Source: three-view drawing plus pictorial views. Frame: mm from the lowest corner of the part. A direction names the side the tool comes from. Give positions to 0.01 mm unless a question says otherwise; leave off trailing zeros. Order: outer loops, then holes, each group sorted by start corner. A loop starts at its lowest first (then second) coordinate and runs counter-clockwise, first axis right, second up. Notation, with made-up numbers: (26, 89.5) -> (49, 89.5) arc R35 ccw to (49, 125.5) -> close; hole circle Ø5 at (-37, 43). An arc over 180 degrees is marked (long way). Answer in a Markdown table with one row per item.
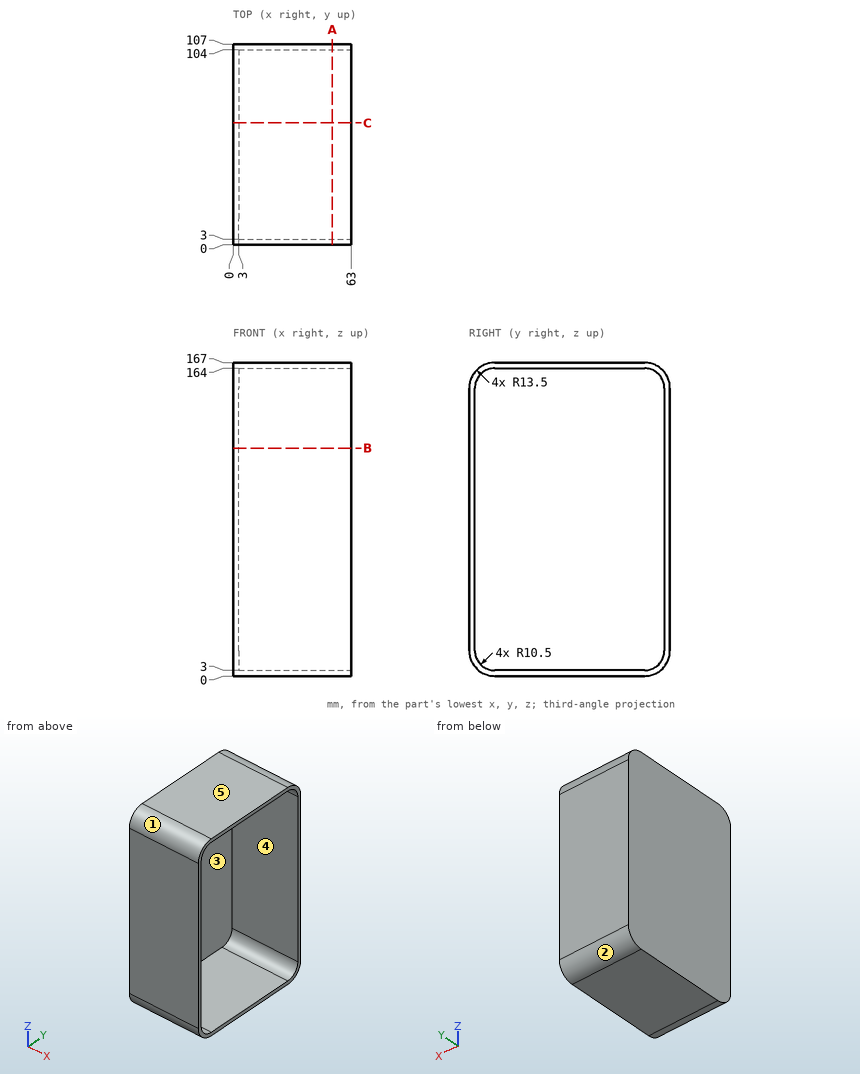
(1) First-contact query: pin 1 Ø2 at (x, z) = (11.5, 148.5) entering from -Y; pin 2 Ø4 at (y, z) = (12, 66.5) entering from +X. Flat tips, straight axial feed; report the tip coordinate or a pass-through.
A:
| item | result |
|---|---|
| pin 1 | stops at y = 0 |
| pin 2 | stops at x = 3 |
(2) Section query B-B (z = 121.5). Return the cut outline in (x, y).
A:
| item | result |
|---|---|
| outline | (0, 0) -> (63, 0) -> (63, 3) -> (3, 3) -> (3, 104) -> (63, 104) -> (63, 107) -> (0, 107) -> close |
(3) Section query A-A (x = 53). Return the cut outline in (y, z).
A:
| item | result |
|---|---|
| outline | (0, 13.5) arc R13.5 ccw to (13.5, 0) -> (93.5, 0) arc R13.5 ccw to (107, 13.5) -> (107, 153.5) arc R13.5 ccw to (93.5, 167) -> (13.5, 167) arc R13.5 ccw to (0, 153.5) -> close; hole (3, 13.5) arc R10.5 ccw to (13.5, 3) -> (93.5, 3) arc R10.5 ccw to (104, 13.5) -> (104, 153.5) arc R10.5 ccw to (93.5, 164) -> (13.5, 164) arc R10.5 ccw to (3, 153.5) -> close |
(4) Access query for the marked faces 4 and 5. Directions: +Z, -Z, +X, -X, +Y, -Y. A direction counts if a zero-diameter tool reaches every point of the face in a straight line with its end or side. Return the directions, or none.
A:
| item | result |
|---|---|
| face 4 | +X |
| face 5 | +Z, +X, -X, +Y, -Y |
(5) Ray query, probe 1 along Y at (x, z) = (33, 21); probe 2 along Z at (x, y) = (23.5, 27.5); probe 3 along X at (y, z) = (94.5, 104). Return the intervals inside material, ascending.
A:
| item | result |
|---|---|
| probe 1 | y = 0 to 3, 104 to 107 |
| probe 2 | z = 0 to 3, 164 to 167 |
| probe 3 | x = 0 to 3 |
(6) Section query C-C (y = 65). Return the cut outline in (x, z), plus the area to 3 significant figures.
A:
| item | result |
|---|---|
| outline | (0, 0) -> (63, 0) -> (63, 3) -> (3, 3) -> (3, 164) -> (63, 164) -> (63, 167) -> (0, 167) -> close |
| area | 861 mm^2 |
(7) Pull-direction query (Y, two-part tool) for the marked faces 1, 2 and 3; classes: +Y half, -Y half, draft (parallel to the pull), parting line (faces both ways), or undercut.
A:
| item | result |
|---|---|
| face 1 | -Y half |
| face 2 | +Y half |
| face 3 | undercut |
